Can you work these out from the model? Positions are in its coordinate system, mm. A direction names the side the tool comes from. Round coordinates to 2 decimals unless told otherwise and drop trailing zeros. Write each loop counter-clockwise with the first axis right and the second up, starting at its lowest first coordinate (ties: lowest second). Pieces come first, ordered by that corner, then holes. Notation, with made-up numbers: (-19, 36) -> (26, 36) arc R27 ccw to (26, 68) -> close; hole circle Ø7 at (62.25, 29). An arc over 180 degrees is marked (long way). Use CSV: the item, a comma, the result in double quotes.
```python
from build123d import *

# Parameters (mm, degrees)
SKETCH1_W                = 17
SKETCH1_H                = 79.3333
SKETCH1_R                = 2.6
SKETCH1_R_2              = 3.985
BOSS_EXTRUDE1_DEPTH      = 17.5
FILLET1_R                = 5
BOSS_EXTRUDE2_DEPTH      = 5.75
BOSS_EXTRUDE2_DEPTH_BACK = 5.75
SKETCH3_R                = 3.985
SKETCH3_R_2              = 2.25
SKETCH2_W                = 40
SKETCH2_H                = 10
SKETCH2_W_2              = 36.666864
SKETCH2_H_2              = 6.45
CUT_EXTRUDE2_DEPTH       = 84.000135475


with BuildPart() as part:
    # Sketch1 → Boss-Extrude1 (new body)
    with BuildSketch(Plane(origin=(0, 0, 0), x_dir=(1, 0, 0), z_dir=(0, 1, 0))):
        with Locations((8.5, 39.66665)):
            Rectangle(SKETCH1_W, SKETCH1_H)
        with Locations(Location((8.5, 10, 0), (0, 0, 270))):
            Circle(SKETCH1_R, mode=Mode.SUBTRACT)
        with Locations(Location((8.5, 60, 0), (0, 0, 270))):
            Circle(SKETCH1_R_2, mode=Mode.SUBTRACT)
        with BuildLine():
            ThreePointArc((7.51420262, 70.4998675), (6.957011868, 69.333201), (7.51420262, 68.1665345))
            ThreePointArc((7.51420262, 68.1665345), (8.457011868, 65.499868), (9.399821116, 68.1665345))
            ThreePointArc((9.399821116, 68.1665345), (9.957011868, 69.333201), (9.399821116, 70.4998675))
            ThreePointArc((9.399821116, 70.4998675), (8.457011868, 73.166534), (7.51420262, 70.4998675))
        make_face(mode=Mode.SUBTRACT)
    extrude(amount=BOSS_EXTRUDE1_DEPTH)

    # Fillet1
    fillet1_edges = [part.edges().sort_by_distance(p)[0] for p in [
        (0, 8.75, -79.3333),
        (17, 8.75, -79.3333),
        (17, 8.75, 0),
        (0, 8.75, 0),
    ]]
    fillet(fillet1_edges, radius=FILLET1_R)

    # Sketch3 → Boss-Extrude2 (add, two sides: drawn at the far end of the back side and taken through both)
    with BuildSketch(Plane(origin=(0, 8.75, 0), x_dir=(1, 0, 0), z_dir=(0, 1, 0)).offset(-BOSS_EXTRUDE2_DEPTH_BACK)):
        with Locations(Location((8.5, 60, 0), (0, 0, 90))):
            Circle(SKETCH3_R)
        with Locations(Location((8.5, 60, 0), (0, 0, 90))):
            Circle(SKETCH3_R_2, mode=Mode.SUBTRACT)
    extrude(amount=BOSS_EXTRUDE2_DEPTH + BOSS_EXTRUDE2_DEPTH_BACK)

    # Sketch2 → Cut-Extrude2 (cut, through all)
    with BuildSketch(Plane(origin=(17, 0, 0), x_dir=(0, 0, -1), z_dir=(1, 0, 0))):
        with Locations((0, 8.75)):
            Rectangle(SKETCH2_W, SKETCH2_H)
        with Locations((79.3333, 8.75)):
            Rectangle(SKETCH2_W_2, SKETCH2_H_2)
    extrude(amount=-CUT_EXTRUDE2_DEPTH, mode=Mode.SUBTRACT)


solid = part.part
```
Q1. Suppose I cut it at A-A (z = -10). Write out the boundary of the cut face in (x, y), and give its area (3 significant figures).
Resolved:
outline,"(0, 0) -> (5.9, 0) -> (5.9, 3.75) -> (0, 3.75) -> close; (0, 13.75) -> (5.9, 13.75) -> (5.9, 17.5) -> (0, 17.5) -> close; (11.1, 0) -> (17, 0) -> (17, 3.75) -> (11.1, 3.75) -> close; (11.1, 13.75) -> (17, 13.75) -> (17, 17.5) -> (11.1, 17.5) -> close"
area,"88.5 mm^2"
Q2. Suppose I cut it at C-C (z = -60). Write out the boundary of the cut face in (x, y) (3 decimals).
Resolved:
outline,"(0, 0) -> (4.515, 0) -> (4.515, 3) -> (6.25, 3) -> (6.25, 14.5) -> (4.515, 14.5) -> (4.515, 17.5) -> (0, 17.5) -> close; (10.75, 3) -> (12.485, 3) -> (12.485, 0) -> (17, 0) -> (17, 17.5) -> (12.485, 17.5) -> (12.485, 14.5) -> (10.75, 14.5) -> close"
Q3. Please list where these lines run through material, in increasing order: probe 1 along Z at (x, y) = (8.5, 1.1) (3 decimals); probe 2 along X at (y, z) = (5.25, -60); probe 3 along X at (y, z) = (1.8, -60) (3 decimals).
Resolved:
probe 1,"z = -79.333 to -73.166, -65.5 to -63.985, -56.015 to -12.6, -7.4 to 0"
probe 2,"x = 0 to 6.25, 10.75 to 17"
probe 3,"x = 0 to 4.515, 12.485 to 17"
Q4. Will these pins go through, and if not, where does the flat tip stop? P1, Ø7, axis at x = 8.5, z = -60, coming from the +Y side; P2, Ø1.9, axis at x = 15, y = 8, coming from the -Z side; P3, Ø1.5, axis at x = 2.5, y = 5.5, coming from the +Z side.
Resolved:
P1,"stops at y = 14.5"
P2,"stops at z = -61"
P3,"stops at z = -20"
Q5. On a 3-axis mill with a long thin cutter (end or side, diameter ignored), from which of +Z, -Z, +X, -X, +Y, -Y can I reach the whole of each face in a straight line? I mean faces 4 (the face through (10, 3, -62)), 5 (the face through (10, 14.5, -62)), 6 (the face through (14, 9, -61)), 7 (the face through (9.957, 2.724, -69.314)), 8 (the face through (15, 16, -1)). Say none if no direction works.
Resolved:
face 4,"-Y"
face 5,"+Y"
face 6,"-Z, +X, -X"
face 7,"+Y, -Y"
face 8,"+Z, +X, +Y, -Y"
Q6. If we mould it in two halves opening along X, with no side actions, what happens to faces 1 (the face through (8.509, 14.699, -73.166)), 2 (the face through (9, 9, -20)), 3 (the face through (0, 9, -39))? For each: released by +X, released by -X, zero draft, split by the parting line, or undercut.
Resolved:
face 1,"undercut"
face 2,"zero draft"
face 3,"released by -X"
Q7. Suppose I cut it at D-D (y = 16.25). Write out the boundary of the cut face in (x, z) (3 decimals).
Resolved:
outline,"(0, -74.333) arc R5 ccw to (5, -79.333) -> (12, -79.333) arc R5 ccw to (17, -74.333) -> (17, -5) arc R5 ccw to (12, 0) -> (5, 0) arc R5 ccw to (0, -5) -> close; hole circle Ø7.97 at (8.5, -60); hole circle Ø5.2 at (8.5, -10); hole (7.514, -70.5) arc R1.5 ccw (long way) to (9.4, -70.5) arc R1.5 ccw to (9.4, -68.167) arc R1.5 ccw (long way) to (7.514, -68.167) arc R1.5 ccw to start"
Q8. Suppose I cut it at B-B (y = 4.75). Write out the boundary of the cut face in (x, z), and give its area (3 significant figures).
Resolved:
outline,"(0, -74.33) arc R5 ccw to (5, -79.33) -> (12, -79.33) arc R5 ccw to (17, -74.33) -> (17, -20) -> (0, -20) -> close; hole circle Ø4.5 at (8.5, -60); hole (7.51, -70.5) arc R1.5 ccw (long way) to (9.4, -70.5) arc R1.5 ccw to (9.4, -68.17) arc R1.5 ccw (long way) to (7.51, -68.17) arc R1.5 ccw to start"
area,"963 mm^2"
